The listing builds one solid part. Answer for the finished solid, in the listing's coordinates (mm). Face numbers are marked on the shaded views. A direction names the side the tool comes from. Give positions to 0.01 mm unless a question says otherwise; leave off trailing zeros. Loops run counter-clockwise (first coordinate to the right, second up) from the corner with the lowest first, then second, coordinate; pieces in that order, holes last.
Item 1: Section A-A, the plane z = 4.75 is taken. Give the vertices of the cut face in (x, y).
Item 2: Section B-B, the plane x = -3.5 is taken. Give the number of separate pieces and of enclosed holes in the cut face, and give its area (3 significant figures).
Item 3: A tool of negligible diameter and unlimited length cuts with its end or side. For the marked faces 1, 2 and 3, from which of +Z, -Z, +X, -X, +Y, -Y can it reach the whole face along a straight path? Write none if from no direction.
Item 4: Consider line 1 along Y through (x, z) = (0, 2); line 2 along Y through (x, z) = (-2, 3.25); line 3 along Y through (x, z) = (-8.5, 5.25). Determine where each line is inside the solid, lowest interval first.
Item 5: The mould has two halves that part along X. Classify the marked faces 4, 5 and 6: pulls with the +X half, pulls with the -X half, needs draft (parallel to the pull), parting line crosses it, or undercut.
Item 6: Each of these flat-tipped pins is pushed along its axis until it touches: pin 1 Ø2 at (x, y) = (-6.5, 19) entering from -Z; pin 2 Ø4 at (y, z) = (1.5, 2) entering from -X; pin 3 Ø1.5 at (x, z) = (10.5, 3) entering from -Y. Where does it stop, or does it pass through?
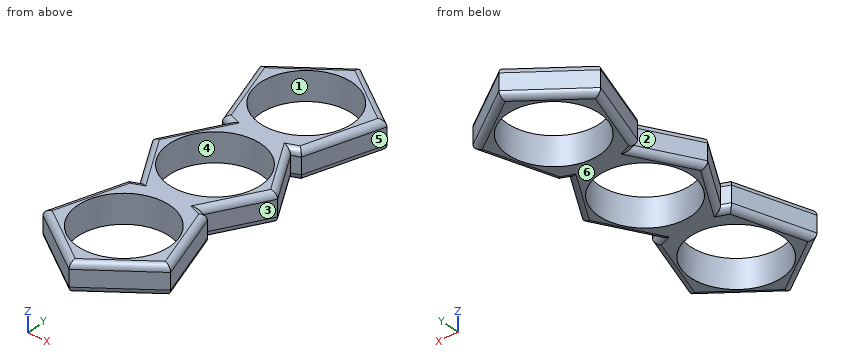
from build123d import *

# Parameters (mm, degrees)
F0_R     = 11.2
F1_DEPTH = 7
F2_R     = 1.5
F3_R     = 1.5


with BuildPart() as f1:
    # F0 (on Top) → F1 (new body)
    with BuildSketch(Plane.XY):
        Polygon((-15.517531, 32.227794), (-9.590361, 13.985842), (-7.621024, 13.2), (-15.242047, 0), (-7.621024, -13.2), (-9.590361, -13.985842), (-15.517531, -32.227794), (0, -43.50194), (15.517531, -32.227794), (9.590361, -13.985842), (7.621024, -13.2), (15.242047, 0), (7.621024, 13.2), (9.590361, 13.985842), (15.517531, 32.227794), (0, 43.50194), align=None)
        with Locations((0, -27.185842)):
            Circle(F0_R, mode=Mode.SUBTRACT)
        Circle(F0_R, mode=Mode.SUBTRACT)
        with Locations((0, 27.185842)):
            Circle(F0_R, mode=Mode.SUBTRACT)
    extrude(amount=F1_DEPTH)

    # F2
    f2_edges = [f1.edges().sort_by_distance(p)[0] for p in [
        (-12.553946, -23.106818, 7),
        (-7.758765, -37.864867, 7),
        (7.758765, -37.864867, 7),
        (12.553946, -23.106818, 7),
        (-8.605692, -13.592921, 7),
        (8.605692, -13.592921, 7),
        (8.605692, 13.592921, 7),
        (-8.605692, 13.592921, 7),
        (-11.431535, 6.6, 7),
        (-11.431535, -6.6, 7),
        (11.431535, -6.6, 7),
        (11.431535, 6.6, 7),
        (12.553946, 23.106818, 7),
        (7.758765, 37.864867, 7),
        (-7.758765, 37.864867, 7),
        (-12.553946, 23.106818, 7),
    ]]
    fillet(f2_edges, radius=F2_R)

    # F3
    f3_edges = [f1.edges().sort_by_distance(p)[0] for p in [
        (-7.758765, -37.864867, 0),
        (-12.553946, -23.106818, 0),
        (12.553946, -23.106818, 0),
        (7.758765, -37.864867, 0),
        (-8.605692, -13.592921, 0),
        (-8.605692, 13.592921, 0),
        (8.605692, 13.592921, 0),
        (8.605692, -13.592921, 0),
        (11.431535, -6.6, 0),
        (-12.553946, 23.106818, 0),
        (-7.758765, 37.864867, 0),
        (7.758765, 37.864867, 0),
        (12.553946, 23.106818, 0),
        (-11.431535, 6.6, 0),
        (-11.431535, -6.6, 0),
        (11.431535, 6.6, 0),
    ]]
    fillet(f3_edges, radius=F3_R)


solid = f1.part
Worked answers:
1. outline: (-15.52, -32.23) - (0, -43.5) - (15.52, -32.23) - (9.59, -13.99) - (7.62, -13.2) - (15.24, 0) - (7.62, 13.2) - (9.59, 13.99) - (15.52, 32.23) - (0, 43.5) - (-15.52, 32.23) - (-9.59, 13.99) - (-7.62, 13.2) - (-15.24, 0) - (-7.62, -13.2) - (-9.59, -13.99) - close; hole circle Ø22.4 at (0, -27.19); hole circle Ø22.4 at (0, 0); hole circle Ø22.4 at (0, 27.19)
2. separate pieces: 4
2. enclosed holes: 0
2. area: 124 mm2
3. face 1: +Z, -Z
3. face 2: +Z, -Z, -X
3. face 3: +Z, -Z, +X
4. line 1: y = -43.5 to -38.39, -15.99 to -11.2, 11.2 to 15.99, 38.39 to 43.5
4. line 2: y = -42.05 to -38.21, -16.17 to -11.02, 11.02 to 16.17, 38.21 to 42.05
4. line 3: y = -37.33 to -34.48, -19.89 to -13.55, -11.68 to -7.29, 7.29 to 11.68, 13.55 to 19.89, 34.48 to 37.33
5. face 4: undercut
5. face 5: pulls with the +X half
5. face 6: needs draft
6. pin 1: stops at z = 0
6. pin 2: stops at x = -15.24
6. pin 3: stops at y = -36.42
